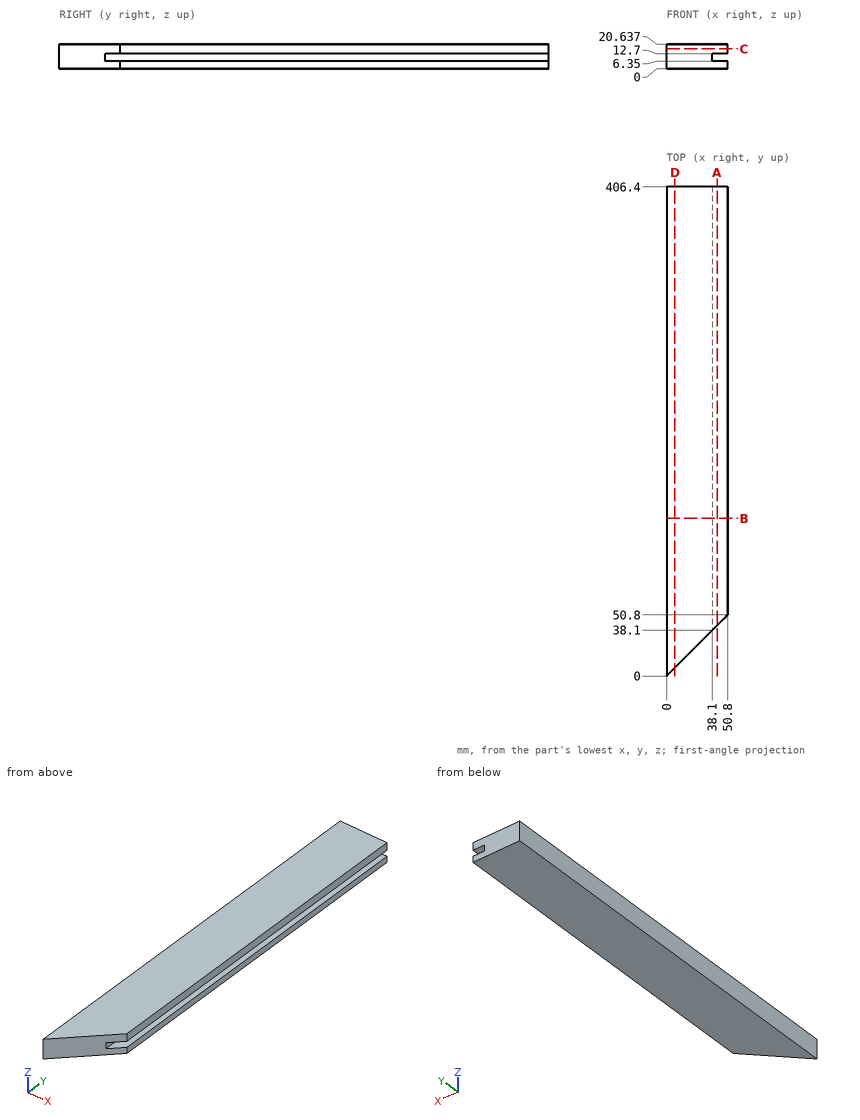
The drawing under review shows one solid part. Ordinate dimensions are in mm from its lowest x, y, z. Coordinates: 2 decimals unless noted, no trailing zeros. Loops run counter-clockwise (first coordinate to the right, second up) from the corner with the lowest first, then second, coordinate; pieces in that order, holes last.
Item 1: Wall thickness on L1, parallel to Z at x = 44.5, y = 140; L2, parallel to X at y = 194.5, z = 10.25; L3, parallel to Y at x = 3, z = 1.25: over which ranges is each line inside the solid? List them lowest first.
Completed:
L1: z = 0 to 6.35, 12.7 to 20.64
L2: x = 0 to 38.1
L3: y = 3 to 406.4
Item 2: Add section B-B (y = 131). Write out the cut boundary in (x, z), and give its area (3 significant figures).
Completed:
outline: (0, 0) - (50.8, 0) - (50.8, 6.35) - (38.1, 6.35) - (38.1, 12.7) - (50.8, 12.7) - (50.8, 20.64) - (0, 20.64) - close
area: 968 mm2
Item 3: Add section C-C (z = 16.5). Write out the cut boundary in (x, y), and give its area (3 significant figures).
Completed:
outline: (0, 0) - (50.8, 50.8) - (50.8, 406.4) - (0, 406.4) - close
area: 19,400 mm2
Item 4: Clearance check with flat-ended pins moving along their axes: pin 1 (3 mm diameter, centred on y = 153.5, z = 10, fed in from -X); pin 2 (3 mm diameter, centred on y = 153.5, z = 8, fed in from +X); pin 3 (5 mm diameter, centred on x = 37, z = 9, fed in from -Y); pin 4 (10 mm diameter, centred on x = 31, z = 16, fed in from -Y). State where each tip first meets the part, or that it passes through.
Completed:
pin 1: stops at x = 0
pin 2: stops at x = 38.1
pin 3: stops at y = 34.5
pin 4: stops at y = 26
Item 5: Add section A-A (x = 42). Write out the cut boundary in (y, z).
Completed:
outline: (42, 0) - (406.4, 0) - (406.4, 6.35) - (42, 6.35) - close; (42, 12.7) - (406.4, 12.7) - (406.4, 20.64) - (42, 20.64) - close
Item 6: Add section D-D (x = 7). Write out the cut boundary in (y, z).
Completed:
outline: (7, 0) - (406.4, 0) - (406.4, 20.64) - (7, 20.64) - close
